Here's how the part is built. I have some questions about the finished solid (model axes, mm). Face numbers are marked on the shaded views. Coordinates: 2 decimals unless noted, no trailing zeros. Loops run counter-clockwise (first coordinate to the right, second up) from the corner with the lowest first, then second, coordinate; pieces in that order, holes last. Notation, with made-up numbers: M 64,14 L 85,14 A18 ccw 85,38 Z; hole C 76.25,66.5 d6. An arc over 180 degrees is marked long. Use one line per item in the form item = value. Start each with the question number.
(1) Imagine slicing it at B-B, the plane y = -20. Please give me the cut outline in (x, z).
(2) Will these pins go through, and if not, where does the flat tip stop? P1, Ø1.4, axis at y = -2, z = 5.5, coming from the -X side; P2, Ø5, axis at x = -32.5, y = 25, coming from the -Z side; P3, Ø0.6, axis at y = -2, z = 5, coming from the +X side.
(3) Thinking about a two-plate mould opening in X: for the marked faces 1 and 2, which applies, +X half, -X half, draft (parallel to the pull), parting line (faces both ways), or undercut?
(4) Imagine slicing it at C-C, the plane y = 29. Please give me the cut outline in (x, z), and give its area (3 significant figures).
(5) Imagine slicing it at A-A, the plane x = 50.8. Please give me the cut outline in (y, z).
(6) Please list where these lines run through material, in increasing order: L1, parallel to Z at x = 50.8, y = -58.25; L2, parallel to X at y = 40, z = -2.5; L3, parallel to X at y = 40.5, z = 2.5.
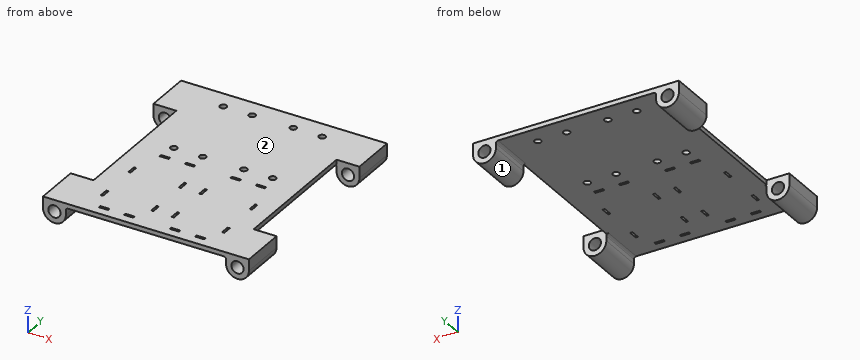
```python
from build123d import *

# Parameters (mm, degrees)
BOSS_EXTRUDE1_DEPTH     = 63.5
SKETCH3_W               = 1.27
SKETCH3_H               = 5.08
CUT_EXTRUDE2_DEPTH      = 87.032540937
LPATTERN1_COUNT         = 2
LPATTERN1_PITCH         = 25.4
LPATTERN1_COUNT_DIR2    = 2
LPATTERN1_PITCH_DIR2    = 27.94
MIRROR1_COPY_1_SKETCH_W = 1.27
MIRROR1_COPY_1_SKETCH_H = 5.08
MIRROR1_COPY_1_DEPTH    = 87.032540937
MIRROR1_COPY_2_SKETCH_W = 1.27
MIRROR1_COPY_2_SKETCH_H = 5.08
MIRROR1_COPY_2_DEPTH    = 87.032540937
MIRROR1_COPY_3_SKETCH_W = 1.27
MIRROR1_COPY_3_SKETCH_H = 5.08
MIRROR1_COPY_3_DEPTH    = 87.032540937
SKETCH5_W               = 5.08
SKETCH5_H               = 1.27
CUT_EXTRUDE3_DEPTH      = 87.032540937
LPATTERN2_COUNT         = 2
LPATTERN2_PITCH         = 13.97
LPATTERN2_COUNT_DIR2    = 2
LPATTERN2_PITCH_DIR2    = 55.88
MIRROR2_COPY_1_SKETCH_W = 5.08
MIRROR2_COPY_1_SKETCH_H = 1.27
MIRROR2_COPY_1_DEPTH    = 87.032540937
MIRROR2_COPY_2_SKETCH_W = 5.08
MIRROR2_COPY_2_SKETCH_H = 1.27
MIRROR2_COPY_2_DEPTH    = 87.032540937
MIRROR2_COPY_3_SKETCH_W = 5.08
MIRROR2_COPY_3_SKETCH_H = 1.27
MIRROR2_COPY_3_DEPTH    = 87.032540937
F_1_0MM_DOWEL_HOLE1_D   = 3.7
LPATTERN3_COUNT         = 2
LPATTERN3_PITCH         = 16.002
LPATTERN3_COUNT_DIR2    = 2
LPATTERN3_PITCH_DIR2    = 45.466
MIRROR3_COPY_1_D        = 3.7
MIRROR3_COPY_2_D        = 3.7
MIRROR3_COPY_3_D        = 3.7
F_1_4_CLEARANCE_HOLE1_D = 6.7564
CUT_EXTRUDE4_DEPTH      = 38.1
FILLET1_R               = 1.27
FILLET2_R               = 1.27


with BuildPart() as part:
    # Sketch1 → Boss-Extrude1 (new, symmetric)
    with BuildSketch(Plane(origin=(0, 0, 0), x_dir=(1, 0, 0), z_dir=(0, 1, 0))):
        with BuildLine():
            Line((0, -6.35), (57.15, -6.35))
            Line((57.15, -6.35), (57.15, 0))
            ThreePointArc((57.15, 0), (50.799999392, 6.349999392), (44.45, -1.216e-06))
            Line((44.45, -1.216e-06), (44.45, -3.81))
            Line((44.45, -3.81), (-44.45, -3.81))
            Line((-44.45, -3.81), (-44.45, 0))
            ThreePointArc((-44.45, 0), (-50.8, 6.35), (-57.15, 0))
            Line((-57.15, 0), (-57.15, -6.35))
            Line((-57.15, -6.35), (0, -6.35))
        make_face()
    extrude(amount=BOSS_EXTRUDE1_DEPTH, both=True)

    # Sketch3 → Cut-Extrude2 (cut, through all)
    with BuildSketch(Plane(origin=(0, 0, 3.81), x_dir=(-1, 0, 0), z_dir=(0, 0, -1))):
        with Locations((5.715, -20.32)):
            Rectangle(SKETCH3_W, SKETCH3_H)
    cut_extrude2 = extrude(amount=-CUT_EXTRUDE2_DEPTH, mode=Mode.SUBTRACT)

    # LPattern1: Cut-Extrude2 2 × 2
    with Locations(*[(-j * LPATTERN1_PITCH_DIR2, -i * LPATTERN1_PITCH, 0) for i in range(LPATTERN1_COUNT) for j in range(LPATTERN1_COUNT_DIR2) if (i, j) != (0, 0)]):
        add(cut_extrude2, mode=Mode.SUBTRACT)

    # Mirror1: Cut-Extrude2 across plane
    add(cut_extrude2.mirror(Plane(origin=(0, 0, 0), x_dir=(0, 0, 1), z_dir=(1, 0, 0))), mode=Mode.SUBTRACT)

    # Mirror1 copy 1 sketch → Mirror1 copy 1 (cut, through all)
    with BuildSketch(Plane(origin=(27.94, 0, 3.81), x_dir=(1, 0, 0), z_dir=(0, 0, -1))):
        with Locations((5.715, 20.32)):
            Rectangle(MIRROR1_COPY_1_SKETCH_W, MIRROR1_COPY_1_SKETCH_H)
    extrude(amount=-MIRROR1_COPY_1_DEPTH, mode=Mode.SUBTRACT)

    # Mirror1 copy 2 sketch → Mirror1 copy 2 (cut, through all)
    with BuildSketch(Plane(origin=(0, -25.4, 3.81), x_dir=(1, 0, 0), z_dir=(0, 0, -1))):
        with Locations((5.715, 20.32)):
            Rectangle(MIRROR1_COPY_2_SKETCH_W, MIRROR1_COPY_2_SKETCH_H)
    extrude(amount=-MIRROR1_COPY_2_DEPTH, mode=Mode.SUBTRACT)

    # Mirror1 copy 3 sketch → Mirror1 copy 3 (cut, through all)
    with BuildSketch(Plane(origin=(27.94, -25.4, 3.81), x_dir=(1, 0, 0), z_dir=(0, 0, -1))):
        with Locations((5.715, 20.32)):
            Rectangle(MIRROR1_COPY_3_SKETCH_W, MIRROR1_COPY_3_SKETCH_H)
    extrude(amount=-MIRROR1_COPY_3_DEPTH, mode=Mode.SUBTRACT)

    # Sketch5 → Cut-Extrude3 (cut, through all)
    with BuildSketch(Plane(origin=(0, 0, 3.81), x_dir=(-1, 0, 0), z_dir=(0, 0, -1))):
        with Locations((12.7, -1.905)):
            Rectangle(SKETCH5_W, SKETCH5_H)
    cut_extrude3 = extrude(amount=-CUT_EXTRUDE3_DEPTH, mode=Mode.SUBTRACT)

    # LPattern2: Cut-Extrude3 2 × 2
    with Locations(*[(-i * LPATTERN2_PITCH, -j * LPATTERN2_PITCH_DIR2, 0) for i in range(LPATTERN2_COUNT) for j in range(LPATTERN2_COUNT_DIR2) if (i, j) != (0, 0)]):
        add(cut_extrude3, mode=Mode.SUBTRACT)

    # Mirror2: Cut-Extrude3 across plane
    add(cut_extrude3.mirror(Plane(origin=(0, 0, 0), x_dir=(0, 0, 1), z_dir=(1, 0, 0))), mode=Mode.SUBTRACT)

    # Mirror2 copy 1 sketch → Mirror2 copy 1 (cut, through all)
    with BuildSketch(Plane(origin=(0, -55.88, 3.81), x_dir=(1, 0, 0), z_dir=(0, 0, -1))):
        with Locations((12.7, 1.905)):
            Rectangle(MIRROR2_COPY_1_SKETCH_W, MIRROR2_COPY_1_SKETCH_H)
    extrude(amount=-MIRROR2_COPY_1_DEPTH, mode=Mode.SUBTRACT)

    # Mirror2 copy 2 sketch → Mirror2 copy 2 (cut, through all)
    with BuildSketch(Plane(origin=(13.97, 0, 3.81), x_dir=(1, 0, 0), z_dir=(0, 0, -1))):
        with Locations((12.7, 1.905)):
            Rectangle(MIRROR2_COPY_2_SKETCH_W, MIRROR2_COPY_2_SKETCH_H)
    extrude(amount=-MIRROR2_COPY_2_DEPTH, mode=Mode.SUBTRACT)

    # Mirror2 copy 3 sketch → Mirror2 copy 3 (cut, through all)
    with BuildSketch(Plane(origin=(13.97, -55.88, 3.81), x_dir=(1, 0, 0), z_dir=(0, 0, -1))):
        with Locations((12.7, 1.905)):
            Rectangle(MIRROR2_COPY_3_SKETCH_W, MIRROR2_COPY_3_SKETCH_H)
    extrude(amount=-MIRROR2_COPY_3_DEPTH, mode=Mode.SUBTRACT)

    # Ø1.0mm Dowel Hole1 (through all)
    with Locations(Plane(origin=(0, 0, 0), x_dir=(1, 0, 0), z_dir=(0, 0, -1))):
        with Locations((-11.43, -7.62)):
            f_1_0mm_dowel_hole1 = Hole(F_1_0MM_DOWEL_HOLE1_D / 2)

    # LPattern3: 1.0mm Dowel Hole1 2 × 2
    with Locations(*[(-i * LPATTERN3_PITCH, j * LPATTERN3_PITCH_DIR2, 0) for i in range(LPATTERN3_COUNT) for j in range(LPATTERN3_COUNT_DIR2) if (i, j) != (0, 0)]):
        add(f_1_0mm_dowel_hole1, mode=Mode.SUBTRACT)

    # Mirror3: Ø1.0mm Dowel Hole1 across plane
    add(f_1_0mm_dowel_hole1.mirror(Plane(origin=(0, 0, 0), x_dir=(0, 0, 1), z_dir=(1, 0, 0))), mode=Mode.SUBTRACT)

    # Mirror3 copy 1 (through all)
    with Locations(Plane(origin=(0, 45.466, 0), x_dir=(-1, 0, 0), z_dir=(0, 0, -1))):
        with Locations((-11.43, 7.62)):
            Hole(MIRROR3_COPY_1_D / 2)

    # Mirror3 copy 2 (through all)
    with Locations(Plane(origin=(16.002, 0, 0), x_dir=(-1, 0, 0), z_dir=(0, 0, -1))):
        with Locations((-11.43, 7.62)):
            Hole(MIRROR3_COPY_2_D / 2)

    # Mirror3 copy 3 (through all)
    with Locations(Plane(origin=(16.002, 45.466, 0), x_dir=(-1, 0, 0), z_dir=(0, 0, -1))):
        with Locations((-11.43, 7.62)):
            Hole(MIRROR3_COPY_3_D / 2)

    # 1/4 Clearance Hole1 (through all)
    with Locations(Plane(origin=(0, 63.5, 0), x_dir=(1, 0, 0), z_dir=(0, 1, 0))):
        with Locations((-50.8, 0)):
            f_1_4_clearance_hole1 = Hole(F_1_4_CLEARANCE_HOLE1_D / 2)

    # Mirror4: 1/4 Clearance Hole1 across plane
    add(f_1_4_clearance_hole1.mirror(Plane(origin=(0, 0, 0), x_dir=(0, 0, 1), z_dir=(1, 0, 0))), mode=Mode.SUBTRACT)

    # Sketch16 → Cut-Extrude4 (cut, symmetric)
    with BuildSketch(Plane(origin=(0, 0, 0), x_dir=(1, 0, 0), z_dir=(0, 1, 0))):
        with BuildLine():
            Line((-57.15, 0), (-57.15, -6.35))
            Line((-57.15, -6.35), (-44.45, -6.35))
            Line((-44.45, -6.35), (-44.45, 0))
            ThreePointArc((-44.45, 0), (-50.8, 6.35), (-57.15, 0))
        make_face()
    cut_extrude4 = extrude(amount=CUT_EXTRUDE4_DEPTH, both=True, mode=Mode.SUBTRACT)

    # Mirror5: Cut-Extrude4 across plane
    add(cut_extrude4.mirror(Plane(origin=(0, 0, 0), x_dir=(0, 0, 1), z_dir=(1, 0, 0))), mode=Mode.SUBTRACT)

    # Fillet1
    fillet1_edges = [part.edges().sort_by_distance(p)[0] for p in [
        (-44.45, 50.8, 3.81),
        (-44.45, -50.8, 3.81),
    ]]
    fillet(fillet1_edges, radius=FILLET1_R)

    # Fillet2
    fillet2_edges = [part.edges().sort_by_distance(p)[0] for p in [
        (44.45, 50.8, 3.81),
        (44.45, -50.8, 3.81),
    ]]
    fillet(fillet2_edges, radius=FILLET2_R)


solid = part.part
```
Answer:
q1.outline = M -44.45,3.81 L -34.29,3.81 L -34.29,6.35 L -44.45,6.35 Z; M -33.02,3.81 L -6.35,3.81 L -6.35,6.35 L -33.02,6.35 Z; M -5.08,3.81 L 5.08,3.81 L 5.08,6.35 L -5.08,6.35 Z; M 6.35,3.81 L 33.02,3.81 L 33.02,6.35 L 6.35,6.35 Z; M 34.29,3.81 L 44.45,3.81 L 44.45,6.35 L 34.29,6.35 Z
q2.P1 = -44.45
q2.P2 = 3.81
q2.P3 = 44.45
q3.face_1 = undercut
q3.face_2 = draft
q4.outline = M -44.45,3.81 L 44.45,3.81 L 44.45,6.35 L -44.45,6.35 Z
q4.area = 226 mm²
q5.outline = M -63.5,-6.35 L -38.1,-6.35 L -38.1,-3.38 L -63.5,-3.38 Z; M -63.5,3.38 L -38.1,3.38 L -38.1,6.35 L -63.5,6.35 Z; M 38.1,-6.35 L 63.5,-6.35 L 63.5,-3.38 L 38.1,-3.38 Z; M 38.1,3.38 L 63.5,3.38 L 63.5,6.35 L 38.1,6.35 Z
q6.L1 = -6.35 to -3.38, 3.38 to 6.35
q6.L2 = -56.64 to -53.07, -48.53 to -44.96, 44.96 to 48.53, 53.07 to 56.64
q6.L3 = -57.15 to -53.07, -48.53 to -44.45, 44.45 to 48.53, 53.07 to 57.15
